Work out the finished part from the listing and answer in its coordinate system (mm). Round coordinates to 2 decimals unless told otherwise and drop trailing zeros. Loops run counter-clockwise (first coordinate to the right, second up) from the corner with the lowest first, then second, coordinate; pieces in that order, holes last.
```python
from build123d import *

# Parameters (mm, degrees)
BOSS_EXTRUDE1_DEPTH = 0.1
SKETCH2_R           = 0.15
BOSS_EXTRUDE2_DEPTH = 1.5
SKETCH3_R           = 2.5
BOSS_EXTRUDE3_DEPTH = 0.3
SKETCH4_R           = 0.1
CUT_EXTRUDE1_DEPTH  = 2.8


with BuildPart() as part:
    # Sketch1 → Boss-Extrude1 (new body)
    with BuildSketch(Plane(origin=(0, 0, 0), x_dir=(1, 0, 0), z_dir=(0, 1, 0))):
        with BuildLine():
            Line((-0.25, 12.763947624), (0.25, 12.763947624))
            Line((0.25, 12.763947624), (0.25, 0.505972083))
            ThreePointArc((0.25, 0.505972083), (0, -0.564364907), (-0.25, 0.505972083))
            Line((-0.25, 0.505972083), (-0.25, 12.763947624))
        make_face()
    extrude(amount=BOSS_EXTRUDE1_DEPTH)

    # Sketch2 → Boss-Extrude2 (add)
    with BuildSketch(Plane.XZ.offset(-0.1)):
        Circle(SKETCH2_R)
    extrude(amount=BOSS_EXTRUDE2_DEPTH)

    # Sketch3 → Boss-Extrude3 (add)
    with BuildSketch(Plane.XZ.offset(1.4)):
        Circle(SKETCH3_R)
    extrude(amount=BOSS_EXTRUDE3_DEPTH)

    # Sketch4 → Cut-Extrude1 (cut, through all)
    with BuildSketch(Plane(origin=(0, 0.1, 0), x_dir=(1, 0, 0), z_dir=(0, 1, 0))):
        Circle(SKETCH4_R)
    extrude(amount=-CUT_EXTRUDE1_DEPTH, mode=Mode.SUBTRACT)


solid = part.part
```
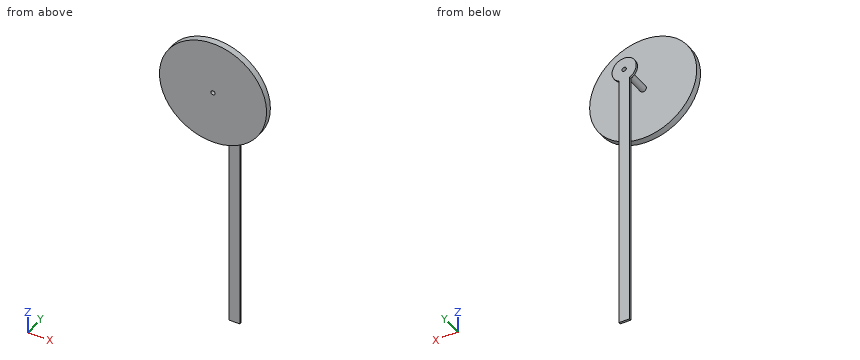
1. Find section C-C (x = 1.7). Write down the section's boundary in (y, z).
Answer key:
outline: (-1.7, -1.83) - (-1.4, -1.83) - (-1.4, 1.83) - (-1.7, 1.83) - close
2. Given pin 1 (0.9 mm diameter, centred on x = 0, z = -5, fed in from -Y), flat-ended and moving along its own axis, determine where the tip first touches the part or whether it passes through.
Answer key:
pin 1: stops at y = 0
3. Consider probe 1 along Y at (x, z) = (1.5, -1); probe 2 along Z at (x, y) = (2, -1.5); probe 3 along X at (y, z) = (-1.6, -0.5). Determine where each line is inside the solid, lowest interval first.
Answer key:
probe 1: y = -1.7 to -1.4
probe 2: z = -1.5 to 1.5
probe 3: x = -2.45 to 2.45
4. Find section A-A (y = -0.7). Write down the section's boundary in (x, z), then the cut area to 3 significant figures.
Answer key:
outline: circle Ø0.3 at (0, 0); hole circle Ø0.2 at (0, 0)
area: 0.0393 mm2
5. Find section B-B (z = -6.5). Write down the section's boundary in (x, y).
Answer key:
outline: (-0.25, 0) - (0.25, 0) - (0.25, 0.1) - (-0.25, 0.1) - close
